For this review, use the dimensioned drawing (mm, ordinates from the lowest corner) and the shaded views. A direction names the side the tool comes from. Round coordinates to 2 decimals unless told otherwise and drop trailing zeros. Write each loop counter-clockwise with the first axis right and the second up, starting at its lowest first coordinate (ties: lowest second). Pieces come first, ordered by that corner, then holes. Notation, with made-up numbers: (-39, -1.5) -> (-23, -1.5) arc R29 ccw to (-23, 33.5) -> close; hole circle Ø10 at (-35.75, 12.5). An arc over 180 degrees is marked (long way). Write each question's results on one line, items separated by ' | '. Start each with the question number.
Item 1: Add section B-B (x = 16.25). State the section outline as (y, z) points.
Item 2: To check wall thickness, follow line 1 along X through (y, z) = (10.25, 1.55); line 2 along Y through (x, z) = (16.25, 1.95); line 3 along X through (y, z) = (5, 2.45). State the ranges of each line that lie inside material, in increasing order.
Item 3: Tool access review of the marked faces 4, 5 and 6: name each direction out of +Z, -Z, +X, -X, +Y, -Y from which nothing blocks a thin tool from reaching the whole face with its end or side.
Item 4: The part is to be moulded in two halves that separate along X. For the marked faces 1, 2 and 3, say which applies: +X half, -X half, draft (parallel to the pull), parting line (faces both ways), or undercut.
Item 5: Add section A-A (x = 10). State the section outline as (y, z) points.
Item 6: Add section D-D (z = 1.95). Count the separate pieces of the cut face and the enclosed holes in it, plus the area to 3 significant figures.
Item 7: Add section C-C (y = 11.25). State the section outline as (x, z) points, plus the area to 3 significant figures.
Item 8: Clearance check with a flat-ended pin moving along its axis: pin 1 (3 mm diameter, centred on x = 3.75, y = 3.75, fed in from +Z). State where the tip first meets the part, or that it passes through.
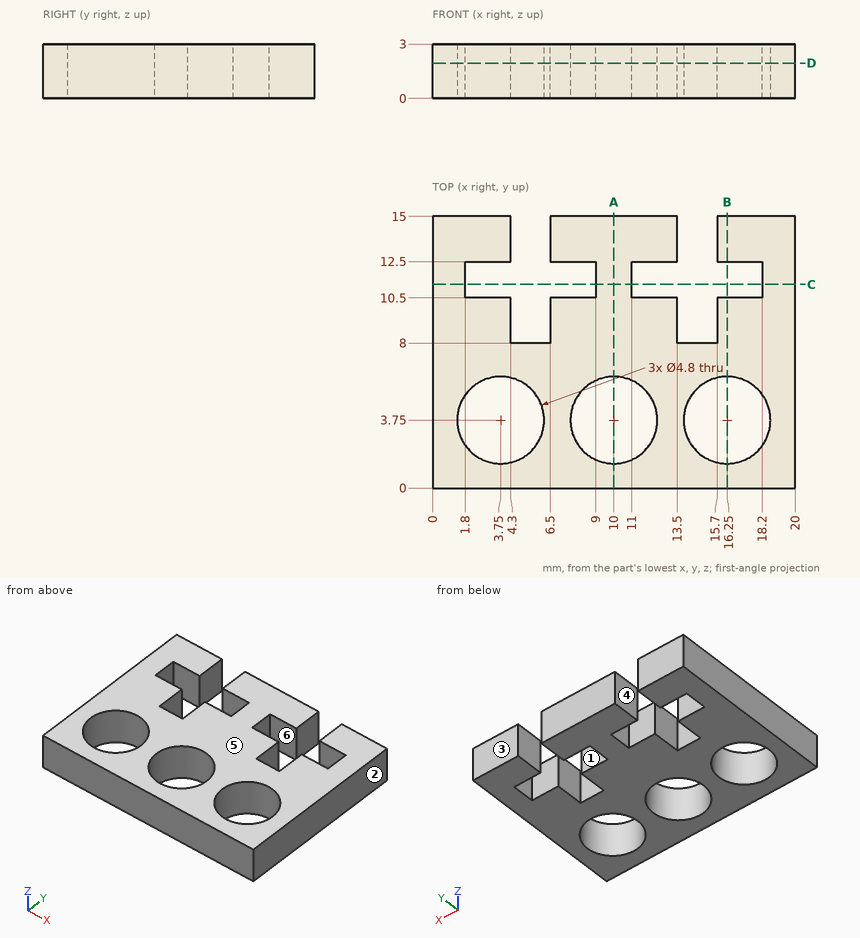
Responses:
1) outline: (0, 0) -> (1.35, 0) -> (1.35, 3) -> (0, 3) -> close; (6.15, 0) -> (10.5, 0) -> (10.5, 3) -> (6.15, 3) -> close; (12.5, 0) -> (15, 0) -> (15, 3) -> (12.5, 3) -> close
2) line 1: x = 0 to 4.3, 6.5 to 13.5, 15.7 to 20 | line 2: y = 0 to 1.35, 6.15 to 10.5, 12.5 to 15 | line 3: x = 0 to 1.7, 5.8 to 7.95, 12.05 to 14.2, 18.3 to 20
3) face 4: +Z, -Z, +Y | face 5: +Z, +X, -X, +Y, -Y | face 6: +Z, -Z
4) face 1: undercut | face 2: +X half | face 3: draft
5) outline: (0, 0) -> (1.35, 0) -> (1.35, 3) -> (0, 3) -> close; (6.15, 0) -> (15, 0) -> (15, 3) -> (6.15, 3) -> close
6) separate pieces: 1 | enclosed holes: 3 | area: 195 mm^2
7) outline: (0, 0) -> (1.8, 0) -> (1.8, 3) -> (0, 3) -> close; (9, 0) -> (11, 0) -> (11, 3) -> (9, 3) -> close; (18.2, 0) -> (20, 0) -> (20, 3) -> (18.2, 3) -> close | area: 16.8 mm^2
8) pin 1: passes through
